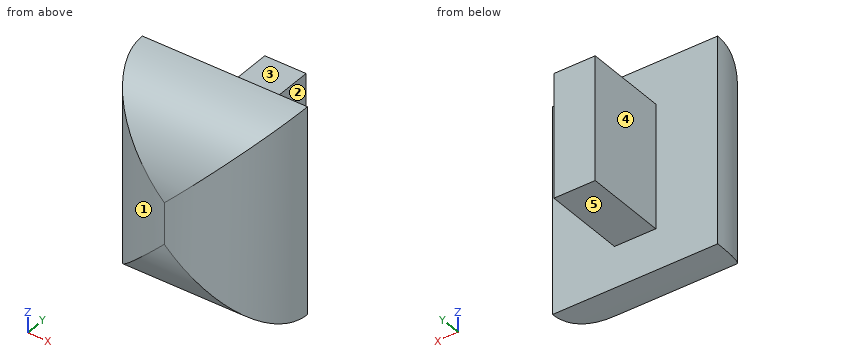
```python
from build123d import *

# Parameters (mm, degrees)
SKETCH1_W           = 6.35
SKETCH1_H           = 7.9375
BOSS_EXTRUDE1_DEPTH = 3.175
SKETCH1_3_W         = 1.5875
SKETCH1_3_H         = 4.7625
BOSS_EXTRUDE2_DEPTH = 3.175
FILLET1_R           = 3.175


with BuildPart() as part:
    # Sketch1 → Boss-Extrude1 (new body)
    with BuildSketch(Plane(origin=(0, 0, 0), x_dir=(1, 0, 0), z_dir=(0, 1, 0))):
        with Locations((3.175, 3.96875)):
            Rectangle(SKETCH1_W, SKETCH1_H)
    extrude(amount=-BOSS_EXTRUDE1_DEPTH)

    # Sketch1<3> → Boss-Extrude2 (add)
    with BuildSketch(Plane(origin=(0, 0, 0), x_dir=(1, 0, 0), z_dir=(0, 1, 0))):
        with Locations((3.175, 3.96875)):
            Rectangle(SKETCH1_3_W, SKETCH1_3_H)
    extrude(amount=BOSS_EXTRUDE2_DEPTH)

    # Fillet1
    fillet1_edges = [part.edges().sort_by_distance(p)[0] for p in [
        (6.35, -3.175, -3.96875),
        (3.175, -3.175, -7.9375),
        (0, -3.175, -3.96875),
        (3.175, -3.175, 0),
    ]]
    fillet(fillet1_edges, radius=FILLET1_R - 0.0001)  # a hair under: the kernel refuses the full size


solid = part.part
```
Could you check a few things on this model? Use its own coordinates, in mm. Face numbers are marked on the shaded views. A direction names the side the tool comes from. Round coordinates to 2 decimals unless told otherwise and drop trailing zeros. Loops run counter-clockwise (first coordinate to the right, second up) from the corner with the lowest first, then second, coordinate; pieces in that order, holes last. Notation, with made-up numbers: (6.5, -20.75) - (16.5, -20.75) arc R15 cw to (16.5, 4.25) - close; hole circle Ø11 at (60, 83). An arc over 180 degrees is marked (long way). Answer in a Markdown table with one row per item. Add a question column.
(1) I'm going to push flat-ended pins straight in: pin 1 (1.7 mm diameter, centred on x = 3, y = 1.5, fed in from +Z); pin 2 (2.5 mm diameter, centred on y = 1.5, z = -5, fed in from -X); pin 3 (1 mm diameter, centred on y = 2, z = -3.5, fed in from +X). Where does each tip first touch, or does it pass through?
(2) If we section it at C-C (y = 1.25): Please give me the cut outline in (x, z).
(3) For the marked faces 1, 2, 3, 4 and 5, which set-ups out of +Z, -Z, +X, -X, +Y, -Y let a thin tool reach every point of the face, with its end or its side?
(4) I need wall thicknesses on line 1 along Z through (x, y) = (3.25, 1.5); line 2 along X through (y, z) = (2.25, -3.75); line 3 along Y through (x, z) = (3.25, -4.25) (3 decimals). Which ranges of each line are inside material? Lowest first, please.
Model answer:
| question | item | result |
|---|---|---|
| 1 | pin 1 | stops at z = -1.59 |
| 1 | pin 2 | stops at x = 2.38 |
| 1 | pin 3 | stops at x = 3.97 |
| 2 | outline | (2.38, -6.35) - (3.97, -6.35) - (3.97, -1.59) - (2.38, -1.59) - close |
| 3 | face 1 | +Z, -Z, -X, -Y |
| 3 | face 2 | +Z, -Z, +X, +Y |
| 3 | face 3 | +Z, +X, -X, +Y |
| 3 | face 4 | +Z, -Z, -X, +Y |
| 3 | face 5 | -Z, +X, -X, +Y |
| 4 | line 1 | z = -6.35 to -1.59 |
| 4 | line 2 | x = 2.38 to 3.97 |
| 4 | line 3 | y = -3.174 to 3.175 |
